```python
from build123d import *

# Parameters (mm, degrees)
SKETCH2_W           = 19.05
SKETCH2_H           = 3.175
BOSS_EXTRUDE1_DEPTH = 3.96875
SKETCH7_R           = 5.49275
BOSS_EXTRUDE2_DEPTH = 0.2778125
CHAMFER1_SIZE       = 0.9525
SKETCH4_OUTSIDE_W   = 107.284
SKETCH4_OUTSIDE_H   = 109.004
SKETCH4_OUTSIDE_R   = 5.55625
CUT_EXTRUDE1_DEPTH  = 25.533595695
CUT_EXTRUDE1_DRAFT  = -60


with BuildPart() as part:
    # Sketch2 → Revolve1 (revolve)
    with BuildSketch(Plane(origin=(0, 0, 0), x_dir=(0, 0, -1), z_dir=(1, 0, 0)), mode=Mode.PRIVATE) as revolve1_sk:
        with Locations((9.525, 1.5875)):
            Rectangle(SKETCH2_W, SKETCH2_H)
    revolve(revolve1_sk.sketch.rotate(Axis((0, 0, 0), (0, 0, -1)), 90), axis=Axis((0, 0, 0), (0, 0, -1)))

    # Sketch3 → Boss-Extrude1 (add)
    with BuildSketch(Plane.XY):
        Polygon((0, 6.415804866), (-5.55625, 3.207902433), (-5.55625, -3.207902433), (0, -6.415804866), (5.55625, -3.207902433), (5.55625, 3.207902433), align=None)
    extrude(amount=BOSS_EXTRUDE1_DEPTH)

    # Sketch7 → Boss-Extrude2 (add)
    with BuildSketch(Plane(origin=(0, 0, 0), x_dir=(-1, 0, 0), z_dir=(0, 0, -1))):
        with Locations(Location((0, 0, 0), (0, 0, 180))):
            Circle(SKETCH7_R)
    extrude(amount=BOSS_EXTRUDE2_DEPTH)

    # Chamfer1
    chamfer1_edges = [part.edges().sort_by_distance(p)[0] for p in [
        (-3.175, 0, -19.05),
    ]]
    chamfer(chamfer1_edges, length=CHAMFER1_SIZE)


with BuildPart() as cut_extrude1_tool:
    # Sketch4 outside → Cut-Extrude1 (with draft: the straight prism first)
    with BuildSketch(Plane.XY.offset(3.96875)):
        Rectangle(SKETCH4_OUTSIDE_W, SKETCH4_OUTSIDE_H)
        Circle(SKETCH4_OUTSIDE_R, mode=Mode.SUBTRACT)
    extrude(amount=-CUT_EXTRUDE1_DEPTH)
    # Cut-Extrude1: the draft: its side faces are tilted about the plane it starts from
    cut_extrude1_sides = [cut_extrude1_tool.faces().sort_by_distance(p)[0] for p in [
        (0, -54.502, -8.798047847),
        (53.642, 0, -8.798047847),
        (0, 54.502, -8.798047847),
        (-53.642, 0, -8.798047847),
        (-5.55625, 0, -8.798047847),
    ]]
    draft(cut_extrude1_sides, Plane.XY.offset(3.96875), CUT_EXTRUDE1_DRAFT)


with BuildPart() as part_1:
    add(part.part)

    # Cut-Extrude1: cut by cut_extrude1_tool
    add(cut_extrude1_tool.part, mode=Mode.SUBTRACT)


solid = part_1.part
```
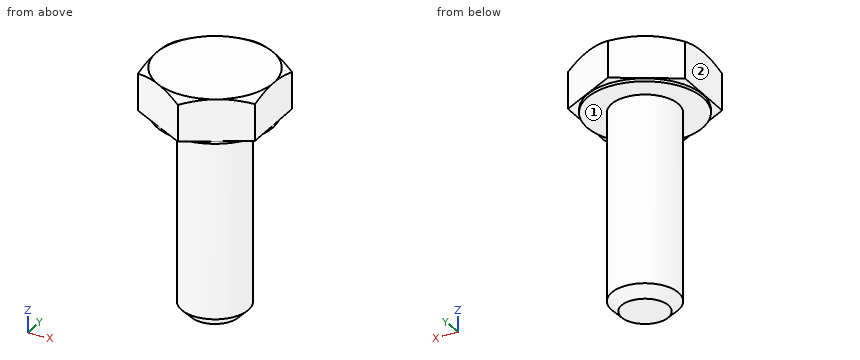
Design review of the part built by this model. Coordinates are the model's own, in mm. Face numbers are marked on the shaded views. A direction names the side the tool comes from. Coordinates: 2 decimals unless noted, no trailing zeros. Order: outer loops, then holes, each group sorted by start corner. A loop starts at its lowest first (then second) coordinate and runs counter-clockwise, first axis right, second up. Notation, with made-up numbers: (61.25, 23) -> (100.25, 23) arc R32 cw to (100.25, 59) -> close; hole circle Ø2 at (66.5, 86). An arc over 180 degrees is marked (long way). One line per item, written item: value. Start each with the question number.
Q1. Tool access review of the marked faces 1 and 2: name each direction out of +Z, -Z, +X, -X, +Y, -Y from which nothing blocks a thin tool from reaching the whole face with its end or side.
Q2. For probe 1 along Z at (x, y) = (-1.5, -5.25); probe 2 along Z at (x, y) = (-0.5, -5.5); probe 3 along X at (y, z) = (-1.75, -2.75), list the stretches that pass through material, from the lowest coordinate up.
Q3. Take a section at A-A, the plane z = 2.5. State the section outline as (x, y) points, then the cut area to 3 significant figures.
Q4. Insertion check: pin 1 Ø6 at (x, z) = (3, -10) entering from +Y (3 decimals); pin 2 Ø3 at (x, z) = (2, -15) entering from -Y. Each pin has a flat end and moves straight along its axis. Give the tip position at first contact, or say it passes through.
Values follow:
1. face 1: -Z
1. face 2: +Z, -Z, -X, +Y, -Y
2. probe 1: z = -0.28 to 3.97
2. probe 2: z = 0 to 3.97
2. probe 3: x = -2.65 to 2.65
3. outline: (-5.56, -3.21) -> (0, -6.42) -> (5.56, -3.21) -> (5.56, 3.21) -> (0, 6.42) -> (-5.56, 3.21) -> close
3. area: 107 mm2
4. pin 1: stops at y = 3.175
4. pin 2: stops at y = -3.14
